Part model, mm, in its own coordinate system. Give positions to 0.01 mm unless a question says otherwise; leave off trailing zeros. Order: outer loops, then holes, each group sorted by start corner. A loop starts at its lowest first (then second) coordinate and runs counter-clockwise, first axis right, second up. Notation, with made-up numbers: M -7.75,-13 L 28.25,-13 A16 cw 28.25,8 Z; hole C 60.5,6 d10. An arc over 180 degrees is marked long. Answer as a JSON object with one key per item and string values.
Autodesk Inventor part; units mm, degrees
ref_plane "YZ Plane" through (0, 0, 0) normal (1, 0, 0) x (0, 1, 0)
ref_plane "XZ Plane" through (0, 0, 0) normal (0, 1, 0) x (-1, 0, 0)
ref_plane "XY Plane" through (0, 0, 0) normal (0, 0, 1) x (1, 0, 0)
sketch "Sketch1" plane through (0, 0, 0) normal (0, 1, 0) x (-1, 0, 0)
  circle A0 centre (0, 7.366) radius 1.75
  circle A1 centre (0, -7.366) radius 1.75
  arc A2 (3.0588, -8.4643) -> (3.0588, 8.4643) centre (0, 0) ccw
  arc A3 (-3.0588, 8.4643) -> (-3.0588, -8.4643) centre (0, 0) ccw
  arc A4 (3.0588, 8.4643) -> (-3.0588, 8.4643) centre (0, 7.366) ccw
  arc A5 (-3.0588, -8.4643) -> (3.0588, -8.4643) centre (0, -7.366) ccw
  point P0 (9, 0)
extrude "Extrusion1" add sketch "Sketch1" along normal blind 5
properties part number "Ball Caster Spacer"
1. Cut at B-B on z = -7. Give the cut face in (x, y), plus the area to 3 significant figures.
Worked answers:
{"outline": "M -5.66,0 L -1.71,0 L -1.71,5 L -5.66,5 Z; M 1.71,0 L 5.66,0 L 5.66,5 L 1.71,5 Z", "area": "39.5 mm^2"}
2. Cut at C-C on y = 0.5. Give the cut face in (x, z), plus the area to 3 significant figures.
Worked answers:
{"outline": "M -3.06,-8.46 A3.25 ccw 3.06,-8.46 A9 ccw 3.06,8.46 A3.25 ccw -3.06,8.46 A9 ccw Z; hole C 0,-7.37 d3.5; hole C 0,7.37 d3.5", "area": "250 mm^2"}
3. Cut at D-D on z = 8. Give the cut face in (x, y), plus the area to 3 significant figures.
Worked answers:
{"outline": "M -4.12,0 L -1.63,0 L -1.63,5 L -4.12,5 Z; M 1.63,0 L 4.12,0 L 4.12,5 L 1.63,5 Z", "area": "24.9 mm^2"}
4. Cut at A-A on x = 0. Give the cut face in (y, z), plus the area to 3 significant figures.
Worked answers:
{"outline": "M 0,-10.62 L 5,-10.62 L 5,-9.12 L 0,-9.12 Z; M 0,-5.62 L 5,-5.62 L 5,5.62 L 0,5.62 Z; M 0,9.12 L 5,9.12 L 5,10.62 L 0,10.62 Z", "area": "71.2 mm^2"}
5. Probe line 1 along Z through (x, y) = (1.5, 1.3); line 2 along Z through (x, y) = (0.25, 3.5); line 3 along X through (y, z) = (1, 7). List the from-to ranges inside material, lowest first.
Worked answers:
{"line 1": "z = -10.25 to -8.27, -6.46 to 6.46, 8.27 to 10.25", "line 2": "z = -10.61 to -9.1, -5.63 to 5.63, 9.1 to 10.61", "line 3": "x = -5.66 to -1.71, 1.71 to 5.66"}
6. Two-plate mould, pull along X, no slides. Class faces 1 (the cylindrical face through (-9, 2, 0)), 2 (the cylindrical face through (0.379, 2.465, -5.658)), 3 (the cylindrical face through (9, 2, 0)): +X half, -X half, draft (parallel to the pull), parting line (faces both ways), or undercut.
Worked answers:
{"face 1": "-X half", "face 2": "undercut", "face 3": "+X half"}
